Read the model definition and answer for the solid it produces. Units are mm, in the model's axes. A direction names the side the tool comes from. Give positions to 0.01 mm unless a question says otherwise; leave off trailing zeros. Order: outer loops, then holes, each group sorted by start corner. A loop starts at its lowest first (then second) coordinate and runs counter-clockwise, first axis right, second up. Notation, with made-up numbers: M 69.25,-4 L 106.25,-4 A11 ccw 106.25,10 Z; hole C -1.75,40.5 d3. An arc over 180 degrees is marked long. One line per item, written item: value. Start each with the question number.
from build123d import *

# Parameters (mm, degrees)
F1_DEPTH = 50
F2_W     = 75
F2_H     = 61.672469
F3_DEPTH = 30
F4_DEPTH = 30
F5_DEPTH = 30
F6_SIZE  = 10


with BuildPart() as f1:
    # F0 (on Front) → F1 (new body)
    with BuildSketch(Plane.XZ):
        Polygon((0, 60), (0, 0), (110, 0), (110, 20), (40, 60), align=None)
    extrude(amount=F1_DEPTH)

    # F2 (on Front) → F3 (cut)
    with BuildSketch(Plane.XZ):
        with Locations((52.5, 29.879423)):
            Rectangle(F2_W, F2_H)
    extrude(amount=-F3_DEPTH, mode=Mode.SUBTRACT)

    # F2 (on Front) → F4 (cut)
    with BuildSketch(Plane.XZ):
        with Locations((52.5, 29.879423)):
            Rectangle(F2_W, F2_H)
    extrude(amount=-F4_DEPTH, mode=Mode.SUBTRACT)

    # F2 (on Front) → F5 (cut)
    with BuildSketch(Plane.XZ):
        with Locations((52.5, 29.879423)):
            Rectangle(F2_W, F2_H)
    extrude(amount=F5_DEPTH, mode=Mode.SUBTRACT)

    # F6
    f6_edges = [f1.edges().sort_by_distance(p)[0] for p in [
        (7.5, 0, 60),
    ]]
    chamfer(f6_edges, length=F6_SIZE)


solid = f1.part
Q1. A tool of negligible diameter and unlimited length cuts with its end or side. For faces 4 (the flat face through (42, -50, 24)), 5 (the flat face through (90, -15, 15)), from which of +Z, -Z, +X, -X, +Y, -Y can it reach the whole face along a straight path? Write none if from no direction.
Q2. Find section D-D, the plane x = 18. Give the vertices of the cut face in (y, z), then the cut area to 3 significant figures.
Q3. Determine the mould class of faces 1 (the flat face through (54.2, -30.2, 0)), 2 (the flat face through (0, -25, 30)), 3 (the flat face through (52, -30, 24)) for opening direction X: released by +X, released by -X, zero draft, split by the parting line, or undercut.
Q4. Each of these flat-tipped pins is pushed along its axis until it touches: pin 1 (1.5 mm diameter, centred on x = 77, z = 18, fed in from +Y); pin 2 (5 mm diameter, centred on x = 65.5, y = -31.5, fed in from +Z); pin 3 (9 mm diameter, centred on y = -9.5, z = 27, fed in from +X) (3 decimals). Where does it stop, or does it pass through?
Q5. Find section A-A, the plane y = -20. Give the vertices of the cut face in (x, z).
Q6. Find section B-B, the plane z = 11. Give the vertices of the cut face in (x, y).
Q7. Find section C-C, the plane y = -43. Give the vertices of the cut face in (x, z).
Q8. Consider probe 1 along X at (y, z) = (-26, 19); probe 2 along Y at (x, z) = (22, 12); probe 3 along X at (y, z) = (-25, 44.5). Determine where each line is inside the solid, lowest interval first.
Evaluation:
1. face 4: +Z, -Z, +X, -X, -Y
1. face 5: +Z, -Z, +Y
2. outline: M -50,0 L -30,0 L -30,60 L -50,60 Z
2. area: 1,200 mm2
3. face 1: zero draft
3. face 2: released by -X
3. face 3: undercut
4. pin 1: y = -30
4. pin 2: z = 46.86
4. pin 3: x = 105.625
5. outline: M 0,0 L 15,0 L 15,60 L 0,60 Z; M 90,0 L 110,0 L 110,20 L 90,31.43 Z
6. outline: M 0,-50 L 110,-50 L 110,0 L 90,0 L 90,-30 L 15,-30 L 15,0 L 0,0 Z
7. outline: M 0,0 L 110,0 L 110,20 L 40,60 L 0,60 Z
8. probe 1: 0 to 15, 90 to 110
8. probe 2: -50 to -30
8. probe 3: 0 to 15
